Autodesk Inventor part; units mm, degrees
ref_plane "YZ Plane" through (0, 0, 0) normal (1, 0, 0) x (0, 1, 0)
ref_plane "XZ Plane" through (0, 0, 0) normal (0, 1, 0) x (-1, 0, 0)
ref_plane "XY Plane" through (0, 0, 0) normal (0, 0, 1) x (1, 0, 0)
sketch "Sketch1" plane through (0, 0, 0) normal (0, 1, 0) x (-1, 0, 0)
  line L0 (0, 0) -> (50, 0)
  line L1 (50, 0) -> (50, -125)
  line L2 (50, -125) -> (0, -125)
  line L3 (0, -125) -> (0, 0)
  dimension "d0" = 50
  dimension "d1" = 125
extrude "Extrusion1" add sketch "Sketch1" along normal blind 10
sketch "Sketch2" plane through (0, 10, 0) normal (0, 1, 0) x (1, 0, 0)
  line L0 (-50, 125) -> (-50, 0)
  line L1 (0, 0) -> (0, 125)
  line L2 (-50, 0) -> (0, 0)
  line L3 (0, 0) -> (0, 20)
  line L4 (0, 20) -> (-50, 20)
  line L5 (-50, 20) -> (-50, 0)
  line L6 (0, 125) -> (-50, 125)
  line L7 (-50, 125) -> (0, 125)
  line L8 (0, 125) -> (0, 105)
  line L9 (0, 105) -> (-50, 105)
  line L10 (-50, 105) -> (-50, 125)
  line L11 (-50, 62.5) -> (0, 62.5)
  line L12 (0, 62.5) -> (0, 72.5)
  line L13 (0, 72.5) -> (-50, 72.5)
  line L14 (-50, 72.5) -> (-50, 62.5)
  line L15 (-50, 62.5) -> (0, 62.5)
  line L16 (0, 62.5) -> (0, 52.5)
  line L17 (0, 52.5) -> (-50, 52.5)
  line L18 (-50, 52.5) -> (-50, 62.5)
  dimension "d4" = 20
  dimension "d5" = 20
  dimension "d6" = 10
  dimension "d7" = 10
extrude "Extrusion2" add sketch "Sketch2" along normal blind 20 contours L6 L1 L9 L0 | L13 L1 L11 L0 | L11 L1 L17 L0 | L4 L1 L2 L0
sketch "Sketch3" plane through (0, 30, 0) normal (0, 1, 0) x (1, 0, 0)
  line L0 (0, 20) -> (0, 52.5)
  line L1 (-50, 0) -> (0, 0)
  line L2 (0, 0) -> (0, 20)
  line L3 (0, 20) -> (-50, 20)
  line L4 (-50, 20) -> (-50, 0)
  line L5 (-50, 52.5) -> (0, 52.5)
  line L6 (0, 72.5) -> (-50, 72.5)
  line L7 (-50, 52.5) -> (0, 52.5)
  line L8 (0, 52.5) -> (0, 72.5)
  line L9 (0, 72.5) -> (-50, 72.5)
  line L10 (-50, 72.5) -> (-50, 52.5)
extrude "Extrusion3" add sketch "Sketch3" along normal blind 100
sketch "Sketch4" plane through (0, 10, -20) normal (0, 0, -1) x (-1, 0, 0)
  line L0 (0, 0) -> (0, 120)
  line L1 (50, 0) -> (50, 120)
  line L2 (0, 120) -> (50, 120)
  line L3 (50, 120) -> (50, 100)
  line L4 (50, 100) -> (0, 100)
  line L5 (0, 100) -> (0, 120)
  line L6 (50, 100) -> (0, 100)
  line L7 (0, 100) -> (0, 70)
  line L8 (0, 70) -> (50, 70)
  line L9 (50, 70) -> (50, 100)
  line L10 (0, 70) -> (50, 70)
  line L11 (50, 70) -> (50, 40)
  line L12 (50, 40) -> (0, 40)
  line L13 (0, 40) -> (0, 70)
  point P0 (0, -10)
  dimension "d12" = 20
  dimension "d13" = 30
  dimension "d14" = 30
extrude "Extrusion4" add sketch "Sketch4" along normal blind 40 contours L0 L8 L1 L12
sketch "Sketch5" plane through (0, 130, 0) normal (0, 1, 0) x (1, 0, 0)
  line L0 (-50, 105) -> (-50, 72.5)
  line L1 (0, 52.5) -> (-50, 52.5)
  line L2 (-50, 52.5) -> (-50, 72.5)
  line L3 (-50, 72.5) -> (0, 72.5)
  line L4 (0, 72.5) -> (0, 52.5)
  point P0 (0, 0)
extrude "Extrusion5" cut sketch "Sketch5" against normal blind 20
sketch "Sketch6" plane through (0, 0, 0) normal (1, 0, 0) x (0, 0, -1)
  point P0 (0, 0)
sketch "Sketch7" plane through (0, 130, 0) normal (0, 1, 0) x (1, 0, 0)
  line L0 (-50, 0) -> (0, 0)
  line L1 (-50, 20) -> (0, 20)
  line L2 (0, 0) -> (-50, 0)
  line L3 (-50, 0) -> (-50, 20)
  line L4 (-50, 20) -> (0, 20)
  line L5 (0, 20) -> (0, 0)
extrude "Extrusion6" add sketch "Sketch7" along normal blind 20
equation "\"BendRadius\" = Thickness"
equation "\"BendReliefWidth\" = Thickness"
equation "\"BendReliefDepth\" = 0.5 * Thickness"
equation "\"CornerReliefSize\" = 4 * Thickness"
equation "\"MinimumRemnant\" = 2 * Thickness"
equation "\"TransitionRadius\" = BendRadius"
equation "\"JacobiRadiusSize\" = BendRadius"
equation "\"GapSize\" = Thickness"
Geometry check sheet. Reference: the model listing, model coordinates, mm. A direction names the side the tool comes from. Coordinates: 2 decimals unless noted, no trailing zeros. Order: outer loops, then holes, each group sorted by start corner. A loop starts at its lowest first (then second) coordinate and runs counter-clockwise, first axis right, second up.
Q1. Depth check by flat-ended pin: pin 1 Ø1.5 at (x, y) = (-29.5, 131) entering from -Z; pin 2 Ø8 at (x, z) = (-13, -44) entering from +Y; pin 3 Ø6 at (x, z) = (-34, -110.5) entering from +Y; pin 4 Ø20 at (x, y) = (-37, 21.5) entering from +Z. Enter the tip coordinate at first touch or a pass-through.
Reply:
pin 1: stops at z = -20
pin 2: stops at y = 80
pin 3: stops at y = 30
pin 4: stops at z = 0
Q2. Sectioned sample at A-A on z = -34.5. Record the cut outline in (x, y).
Reply:
outline: (-50, 0) - (0, 0) - (0, 10) - (-50, 10) - close; (-50, 50) - (0, 50) - (0, 80) - (-50, 80) - close
Q3. Tool access check on faces 5 (the face through (-25, 80, -36)), 6 (the face through (-25, 30, -115)), 7 (the face through (-25, 10, -36)), 8 (the face through (-50, 57, -34)). Record the directions out of +Z, -Z, +X, -X, +Y, -Y that give a thin tool (end or side, any length) a straight path to the whole face; none if there is none.
Reply:
face 5: +X, -X, +Y
face 6: -Z, +X, -X, +Y
face 7: +X, -X
face 8: +Z, -Z, -X, +Y, -Y
Q4. Sectioned sample at D-D on y = 25. Record the cut outline in (x, z).
Reply:
outline: (-50, -125) - (0, -125) - (0, -105) - (-50, -105) - close; (-50, -72.5) - (0, -72.5) - (0, -52.5) - (-50, -52.5) - close; (-50, -20) - (0, -20) - (0, 0) - (-50, 0) - close
Q5. Draft check along Y on faces 1 (the face through (-25, 30, -20)), 2 (the face through (-25, 110, -63)), 3 (the face through (-25, 50, -36)), 4 (the face through (0, 57, -49)). Enter one of: released by +Y, released by -Y, zero draft, split by the parting line, or undercut.
Reply:
face 1: undercut
face 2: released by +Y
face 3: undercut
face 4: zero draft
Q6. Thickness scan on probe 1 along Z at (x, y) = (-12.5, 26); probe 2 along Y at (x, z) = (-7, -32.5); probe 3 along Z at (x, y) = (-43, 107). Record the ranges inside material, lowest first.
Reply:
probe 1: z = -125 to -105, -72.5 to -52.5, -20 to 0
probe 2: y = 0 to 10, 50 to 80
probe 3: z = -72.5 to -52.5, -20 to 0
Q7. Sectioned sample at C-C on x = -14. Record the cut outline in (y, z).
Reply:
outline: (0, -125) - (30, -125) - (30, -105) - (10, -105) - (10, -72.5) - (110, -72.5) - (110, -52.5) - (80, -52.5) - (80, -20) - (150, -20) - (150, 0) - (0, 0) - close; hole (10, -52.5) - (50, -52.5) - (50, -20) - (10, -20) - close
Q8. Sectioned sample at B-B on y = 82. Record the cut outline in (x, z), and give its area (3 significant figures).
Reply:
outline: (-50, -72.5) - (0, -72.5) - (0, -52.5) - (-50, -52.5) - close; (-50, -20) - (0, -20) - (0, 0) - (-50, 0) - close
area: 2,000 mm2
